Could you check a few things on this drawing? It's one solid part, dimensions in mm from its lowest x, y, z. Round coordinates to 2 decimals unless told otherwise and drop trailing zeros. Write each loop counter-clockwise with the first axis right and the second up, starting at its lowest first coordinate (ties: lowest second). Pieces come first, ordered by that corner, then holes. Notation, with made-up numbers: (51, 41.5) -> (107, 41.5) arc R23 ccw to (107, 61.5) -> close; hole circle Ø2 at (84, 29.25). An arc over 180 degrees is marked (long way). Answer in a Markdown table with one row per item.
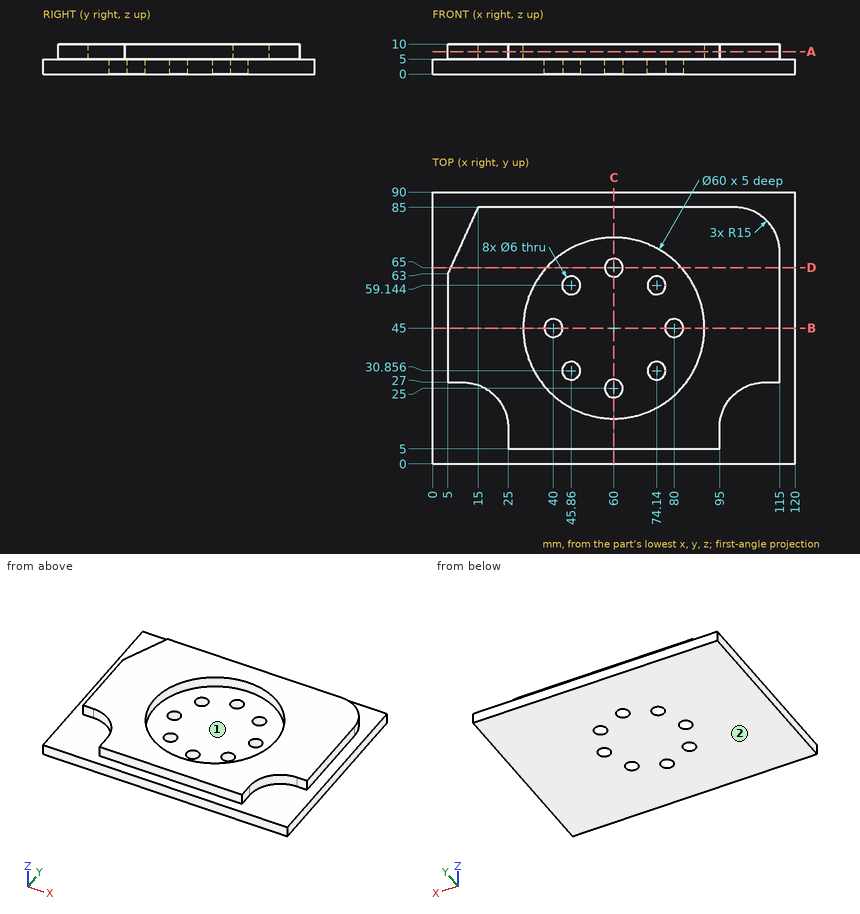
1) Imagine slicing it at D-D, the plane y = 65. Please give me the cut outline in (x, z), plus the area to 3 significant figures.
Findings:
| item | result |
|---|---|
| outline | (0, 0) -> (57, 0) -> (57, 5) -> (37.64, 5) -> (37.64, 10) -> (5.91, 10) -> (5.91, 5) -> (0, 5) -> close; (63, 0) -> (120, 0) -> (120, 5) -> (115, 5) -> (115, 10) -> (82.36, 10) -> (82.36, 5) -> (63, 5) -> close |
| area | 892 mm^2 |
2) Imagine slicing it at B-B, the plane y = 45. Please give me the cut outline in (x, z).
Findings:
| item | result |
|---|---|
| outline | (0, 0) -> (37, 0) -> (37, 5) -> (30, 5) -> (30, 10) -> (5, 10) -> (5, 5) -> (0, 5) -> close; (43, 0) -> (77, 0) -> (77, 5) -> (43, 5) -> close; (83, 0) -> (120, 0) -> (120, 5) -> (115, 5) -> (115, 10) -> (90, 10) -> (90, 5) -> (83, 5) -> close |
3) For pin 1 (9.5 mm diameter, centred on x = 74.14, y = 59.14, fed in from +Z); pin 2 (5.5 mm diameter, centred on x = 72.5, z = 8, fed in from +Y); pin 3 (2.5 mm diameter, centred on x = 7, z = 8, fed in from -Y), each with a flat end and sliding along its axis, tell me the tip position at first contact or that it passes through.
Findings:
| item | result |
|---|---|
| pin 1 | stops at z = 5 |
| pin 2 | stops at y = 85 |
| pin 3 | stops at y = 27 |
4) Please list where these lines run through material, in increasing order: line 1 (Y direction, x = 74.14, z = 2.65); line 2 (Y direction, x = 80, z = 1.9); line 3 (X direction, y = 33.5, z = 3) (1 decimal).
Findings:
| item | result |
|---|---|
| line 1 | y = 0 to 27.86, 33.86 to 56.14, 62.14 to 90 |
| line 2 | y = 0 to 42, 48 to 90 |
| line 3 | x = 0 to 44.4, 47.3 to 72.7, 75.6 to 120 |
5) Thinking about a two-plate mould opening in X: for the marked faces 1 and 2, which applies, +X half, -X half, draft (parallel to the pull), parting line (faces both ways), or undercut?
Findings:
| item | result |
|---|---|
| face 1 | undercut |
| face 2 | draft |
6) Imagine slicing it at A-A, the plane z = 7.5. Please give me the cut outline in (x, y).
Findings:
| item | result |
|---|---|
| outline | (5, 27) -> (10, 27) arc R15 cw to (25, 12) -> (25, 5) -> (95, 5) -> (95, 12) arc R15 cw to (110, 27) -> (115, 27) -> (115, 70) arc R15 ccw to (100, 85) -> (15, 85) -> (5, 63) -> close; hole circle Ø60 at (60, 45) |
7) Imagine slicing it at C-C, the plane x = 60. Please give me the cut outline in (y, z), plus the area to 3 significant figures.
Findings:
| item | result |
|---|---|
| outline | (0, 0) -> (22, 0) -> (22, 5) -> (15, 5) -> (15, 10) -> (5, 10) -> (5, 5) -> (0, 5) -> close; (28, 0) -> (62, 0) -> (62, 5) -> (28, 5) -> close; (68, 0) -> (90, 0) -> (90, 5) -> (85, 5) -> (85, 10) -> (75, 10) -> (75, 5) -> (68, 5) -> close |
| area | 490 mm^2 |
